The listing builds one solid part. Answer for the finished solid, in the listing's coordinates (mm). A direction names the side the tool comes from. Give positions to 0.01 mm unless a question says otherwise; leave off trailing zeros. Order: outer loops, then holes, each group sorted by start corner. A loop starts at its lowest first (then second) coordinate and runs counter-clockwise, first axis right, second up.
```python
from build123d import *

# Parameters (mm, degrees)
SKETCH1_R           = 25.4
BOSS_EXTRUDE1_DEPTH = 35.052
SKETCH2_R           = 20.066
BOSS_EXTRUDE2_DEPTH = 59.69
SKETCH3_R           = 3.175
BOSS_EXTRUDE3_DEPTH = 26.416


with BuildPart() as part:
    # Sketch1 → Boss-Extrude1 (new body)
    with BuildSketch(Plane.XY):
        Circle(SKETCH1_R)
    extrude(amount=BOSS_EXTRUDE1_DEPTH)

    # Sketch2 → Boss-Extrude2 (add)
    with BuildSketch(Plane.XY.offset(35.052)):
        with Locations(Location((0, 0, 0), (0, 0, 180))):
            Circle(SKETCH2_R)
    extrude(amount=BOSS_EXTRUDE2_DEPTH)

    # Sketch3 → Boss-Extrude3 (add)
    with BuildSketch(Plane(origin=(0, 0, 0), x_dir=(-1, 0, 0), z_dir=(0, 0, -1))):
        with Locations(Location((0, -4.7625, 0), (0, 0, 180))):
            Circle(SKETCH3_R)
    extrude(amount=BOSS_EXTRUDE3_DEPTH)


solid = part.part
```
1) Given P1, Ø6, axis at x = 8.5, z = -2, coming from the +Y side; P2, Ø15, axis at x = -4, y = -1, coming from the -Z side; P3, Ø3, axis at y = 15, z = 25.5, coming from the +X side; P4, Ø5, axis at x = 18, z = 5, coming from the -Y side, each flat-ended and moving along its own axis, determine where each tip first touches the part or whether it passes through.
Geometry says:
P1: stops at y = 24.62
P2: stops at z = -26.42
P3: stops at x = 21.52
P4: stops at y = -20.12
2) A tool of negligible diameter and unlimited length cuts with its end or side. For faces 1 (the cylindrical face through (-5.506, -24.796, 17.281)), 2 (the flat face through (19, 8, 35.052)), from which of +Z, -Z, +X, -X, +Y, -Y can it reach the whole face along a straight path? Write none if from no direction.
Geometry says:
face 1: +Z, -Z
face 2: +Z
3) Find section C-C (z = 72). Write down the section's boundary in (x, y), then the cut area to 3 significant figures.
Geometry says:
outline: circle Ø40.13 at (0, 0)
area: 1,260 mm2
4) Straight lines are drawn through the part: probe 1 along Z at (x, y) = (10, 2); probe 2 along Z at (x, y) = (14, -17.5); probe 3 along Y at (x, z) = (-1, 14). For each, find the intervals that lie inside material, in ascending order.
Geometry says:
probe 1: z = 0 to 94.74
probe 2: z = 0 to 35.05
probe 3: y = -25.38 to 25.38
5) Find section B-B (y = 0). Write down the section's boundary in (x, z), then the cut area to 3 significant figures.
Geometry says:
outline: (-25.4, 0) - (25.4, 0) - (25.4, 35.05) - (20.07, 35.05) - (20.07, 94.74) - (-20.07, 94.74) - (-20.07, 35.05) - (-25.4, 35.05) - close
area: 4,180 mm2
6) Find section D-D (x = 7.5). Write down the section's boundary in (y, z).
Geometry says:
outline: (-24.27, 0) - (24.27, 0) - (24.27, 35.05) - (18.61, 35.05) - (18.61, 94.74) - (-18.61, 94.74) - (-18.61, 35.05) - (-24.27, 35.05) - close
7) Find section A-A (x = 0). Write down the section's boundary in (y, z).
Geometry says:
outline: (-25.4, 0) - (-7.94, 0) - (-7.94, -26.42) - (-1.59, -26.42) - (-1.59, 0) - (25.4, 0) - (25.4, 35.05) - (20.07, 35.05) - (20.07, 94.74) - (-20.07, 94.74) - (-20.07, 35.05) - (-25.4, 35.05) - close
8) For a pull along Z with two mould halves and no side action, classify faces 3 (the cylindrical face through (-0.688, -1.663, -13.023)), 4 (the flat face through (0, 0, 0)), 5 (the flat face through (0, 0, 94.742)) as +Z half, -Z half, draft (parallel to the pull), parting line (faces both ways), or undercut.
Geometry says:
face 3: draft
face 4: -Z half
face 5: +Z half
